from build123d import *

# Parameters (mm, degrees)
F1_DEPTH = 5.55625
F2_R     = 1.1303
F2_R_2   = 1.2192
F3_DEPTH = 25.4
F4_R     = 2.778115


# Not quite as in the source:
# - a fillet or chamfer is up to 0.001 mm smaller than in the source, because OpenCascade refuses the exact size


with BuildPart() as f1:
    # F0 (on Front) → F1 (new body)
    with BuildSketch(Plane.XZ):
        Polygon((27.4460728326, 28.3541232628), (19.5085728326, 28.3541232628), (19.5085728326, 26.7666232628), (25.8585728326, 26.7666232628), (25.8585728326, 24.3853732628), (19.5085728326, 24.3853732628), (19.5085728326, 22.7978732628), (27.4460728326, 22.7978732628), align=None)
        with BuildLine():
            ThreePointArc((33.0023228326, 28.3541232628), (30.2241978326, 26.7162135284), (27.4460728326, 28.3541232628))
            Line((27.4460728326, 28.3541232628), (27.4460728326, 22.7978732628))
            ThreePointArc((27.4460728326, 22.7978732628), (30.2241978326, 24.4357829973), (33.0023228326, 22.7978732628))
            Line((33.0023228326, 22.7978732628), (33.0023228326, 28.3541232628))
        make_face()
        Polygon((40.9398228326, 28.3541232628), (33.0023228326, 28.3541232628), (33.0023228326, 22.7978732628), (40.9398228326, 22.7978732628), (40.9398228326, 24.3853732628), (34.5898228326, 24.3853732628), (34.5898228326, 26.7666232628), (40.9398228326, 26.7666232628), align=None)
    extrude(amount=F1_DEPTH)

    # F2 (on face) → F3 (cut)
    with BuildSketch(Plane.XY.offset(28.3541232628)):
        with Locations((22.2866978326, -2.778125)):
            Circle(F2_R)
        with Locations((38.1616978326, -2.778125)):
            Circle(F2_R_2)
    extrude(amount=-F3_DEPTH, mode=Mode.SUBTRACT)

    # F4 (radius 2.778125 in the source; OpenCascade refuses exactly that, so slightly less here)
    f4_edges = [f1.edges().sort_by_distance(p)[0] for p in [
        (19.508573, 0, 23.591623),
        (19.508573, 0, 27.560373),
        (19.508573, -5.55625, 27.560373),
        (19.508573, -5.55625, 23.591623),
        (40.939823, 0, 23.591623),
        (40.939823, 0, 27.560373),
        (40.939823, -5.55625, 23.591623),
        (40.939823, -5.55625, 27.560373),
    ]]
    fillet(f4_edges, radius=F4_R)


solid = f1.part
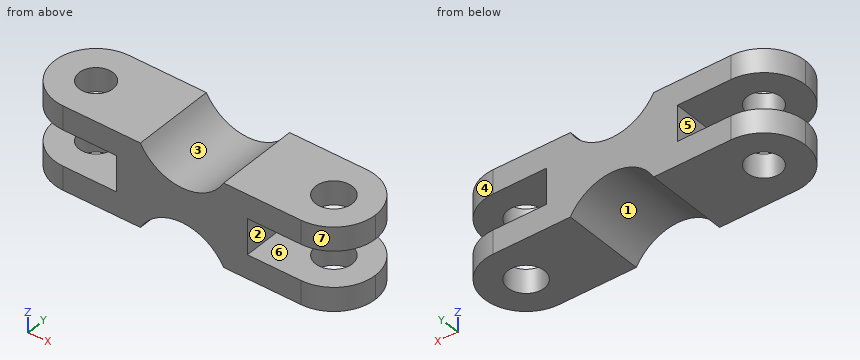
Geometry check sheet. Reference: the model listing, model coordinates, mm. Face numbers are marked on the shaded views. A direction names the side the tool comes from. Give positions to 0.01 mm unless a question says otherwise; leave off trailing zeros. Write each loop counter-clockwise with the first axis right and the second up, starting at its lowest first coordinate (ties: lowest second). Pieces come first, ordered by that corner, then holes. Notation, with made-up numbers: M -30.5,44.25 L -26.5,44.25 A31 cw -26.5,80.25 Z; hole C 47,1.5 d2. An arc over 180 degrees is marked long. Answer as CSV lines item,"result". Start each with the question number.
Q1. Go/stop test with flat-tipped pins: pin 1 (0.7 mm diameter, centred on y = -2.5, z = 26, fed in from -X); pin 2 (2 mm diameter, centred on y = -3, z = 25.5, fed in from +X). Record where each tip stops, or that it passes through.
Q2. Tool access check on the marked faces 5, 6 and 7. Record the directions out of +Z, -Z, +X, -X, +Y, -Y that give a thin tool (end or side, any length) a straight path to the whole face; none if there is none.
Q3. Release check for a two-part mould opening along Z. For the marked faces 1, 2, 3 and 4 record: pulls with the +Z half, pulls with the -Z half, needs draft (parallel to the pull), parting line crosses it, or undercut.
Q4. Section check D-D, the plane x = 37.75. Record the cut outline in (y, z).
Q5. Section check A-A, the plane z = 23.9. Give the number of separate pieces and of enclosed holes in the cut face, then the cut area to 3 significant figures.
Q6. Material ranges on L1, parallel to Z at x = 35, y = -0.45; L2, parallel to X at y = -3, z = 24 (3 decimals); L3, parallel to Y at x = 38.25, z = 23.95, recorded low to high.
Q7. Section check B-B, the plane x = 35.25. Record the cut outline in (y, z), then the cut area to 3 significant figures.
Geometry says:
1,pin 1,"x = 25.86"
1,pin 2,"x = 34.59"
2,face 5,"-X, +Y, -Y"
2,face 6,"+X, +Y, -Y"
2,face 7,"+Z, -Z, +X, -Y"
3,face 1,"pulls with the -Z half"
3,face 2,"undercut"
3,face 3,"pulls with the +Z half"
3,face 4,"needs draft"
4,outline,"M -5.56,22.8 L -3.93,22.8 L -3.93,24.39 L -5.56,24.39 Z; M -5.56,26.77 L -3.93,26.77 L -3.93,28.35 L -5.56,28.35 Z; M -1.63,22.8 L 0,22.8 L 0,24.39 L -1.63,24.39 Z; M -1.63,26.77 L 0,26.77 L 0,28.35 L -1.63,28.35 Z"
5,separate pieces,"2"
5,enclosed holes,"2"
5,area,"84.2 mm^2"
6,L1,"22.8 to 24.39, 26.77 to 28.35"
6,L2,"19.517 to 21.178, 23.395 to 28.619, 31.83 to 36.963, 39.361 to 40.931"
6,L3,"-5.55 to -3.99, -1.56 to 0"
7,outline,"M -5.56,22.8 L 0,22.8 L 0,24.39 L -5.56,24.39 Z; M -5.56,26.77 L 0,26.77 L 0,28.35 L -5.56,28.35 Z"
7,area,"17.6 mm^2"
